from build123d import *

# Parameters (mm, degrees)
F1_DEPTH = 2
F3_DEPTH = 6
F4_W     = 8.5
F4_H     = 26
F5_DEPTH = 6


with BuildPart() as f1:
    # F0 (on Front) → F1 (new body)
    with BuildSketch(Plane.XZ):
        with BuildLine():
            Line((-10, -10), (-10, 0))
            Line((-10, 0), (-10, 18))
            Line((-10, 18), (-11.548888, 17.814133))
            ThreePointArc((-11.548888, 17.814133), (-19.724596, 13.534146), (-23, 4.906735))
            Line((-23, 4.906735), (-23, -10))
            Line((-23, -10), (-10, -10))
        make_face()
        Polygon((-10, 0), (0, 0), (40, 0), (40, 24), (-10, 18), align=None)
    extrude(amount=-F1_DEPTH)

    # F2 (on face) → F3 (join)
    with BuildSketch(Plane.XZ):
        with BuildLine():
            Line((0, 2), (38, 2))
            Line((38, 2), (38, 21.745651))
            Line((38, 21.745651), (-11.310597, 15.82838))
            ThreePointArc((-11.310597, 15.82838), (-18.228504, 12.206852), (-21, 4.906735))
            Line((-21, 4.906735), (-21, -8))
            Line((-21, -8), (-12, -8))
            Line((-12, -8), (-12, 2))
            Line((-12, 2), (0, 2))
        make_face()
    extrude(amount=F3_DEPTH)

    # F4 (on face) → F5 (cut)
    with BuildSketch(Plane.XZ.offset(6)):
        with Locations((27.75, 9.903788)):
            Rectangle(F4_W, F4_H)
    extrude(amount=-F5_DEPTH, mode=Mode.SUBTRACT)


solid = f1.part
Work out the finished part from the listing and answer in its coordinate system (mm). A direction names the side the tool comes from. Round coordinates to 2 decimals unless told otherwise and drop trailing zeros. Order: outer loops, then holes, each group sorted by start corner. A loop starts at its lowest first (then second) coordinate and runs counter-clockwise, first axis right, second up. Notation, with made-up numbers: M 80.25,-25.75 L 88.25,-25.75 A22 cw 88.25,9.25 Z; hole C -4.5,-18.5 d8. An arc over 180 degrees is marked long. Put each result on its own line as item: value. Start each with the question number.
Q1. Straight lines are drawn through the part: L1, parallel to Y at x = 34, z = 1.5; L2, parallel to X at y = -3.5, z = -4.5; L3, parallel to X at y = -3.25, z = 12. For each, find the intervals that lie inside material, in ascending order. Write a range as [from, to].
Q2. Flat-ended cylindrical pins translate along their axes: pin 1 (1.5 mm diameter, centred on y = 1, z = 17.5, fed in from -X); pin 2 (3 mm diameter, centred on x = -2, y = -2, fed in from -Z); pin 3 (3 mm diameter, centred on x = -18, y = -3.5, fed in from -Z). Find the tip coordinate at first contact, or state that the pin passes through.
Q3. Section A-A, the plane y = -4 is taken. Write down the section's boundary in (x, z).
Q4. Section D-D, the plane z = 14 is taken. Write down the section's boundary in (x, y), and give its area (3 significant figures).
Q5. A tool of negligible diameter and unlimited length cuts with its end or side. For faces 1 (the flat face through (-17, -3, -8)), 2 (the flat face through (6.338, -2.958, 17.946)), 3 (the flat face through (6, -3, 2)), 4 (the flat face through (15, 1, 0)), from which of +Z, -Z, +X, -X, +Y, -Y can it reach the whole face along a straight path? Write none if from no direction.
Q6. Section B-B, the plane x = 9 is taken. Write down the section's boundary in (y, z).
Q7. For a pull along X with two mould halves and no side action, classify faces 5 (the flat face through (35, -6, 12)), 6 (the flat face through (38, -3, 12)), 7 (the flat face through (32, -3, 11)) as pulls with the +X half, pulls with the -X half, needs draft (parallel to the pull), parting line crosses it, or undercut.
Q8. Section C-C, the plane y = 1.25 is taken. Write down the section's boundary in (x, z), and give its area (3 significant figures).
Findings below:
1. L1: y = [0, 2]
1. L2: x = [-21, -12]
1. L3: x = [-18.41, 23.5], [32, 38]
2. pin 1: stops at x = -15.36
2. pin 2: stops at z = 2
2. pin 3: stops at z = -8
3. outline: M -21,-8 L -12,-8 L -12,2 L 23.5,2 L 23.5,20.01 L -11.31,15.83 A11 ccw -21,4.91 Z; M 32,2 L 38,2 L 38,21.75 L 32,21.03 Z
4. outline: M -19.29,0 L -16.19,0 L -16.19,-6 L 23.5,-6 L 23.5,0 L 32,0 L 32,-6 L 38,-6 L 38,0 L 40,0 L 40,2 L -19.29,2 Z
4. area: 393 mm^2
5. face 1: -Z, +X, -X, -Y
5. face 2: +Z, -X, -Y
5. face 3: -Z, +X, -Y
5. face 4: -Z, +X, +Y, -Y
6. outline: M -6,2 L 0,2 L 0,0 L 2,0 L 2,20.28 L 0,20.28 L 0,18.27 L -6,18.27 Z
7. face 5: needs draft
7. face 6: pulls with the +X half
7. face 7: undercut
8. outline: M -23,-10 L -10,-10 L -10,0 L 40,0 L 40,24 L -10,18 L -11.55,17.81 A13 ccw -23,4.91 Z
8. area: 1,380 mm^2
